from build123d import *

# Parameters (mm, degrees)
SKETCH1_R           = 11
BOSS_EXTRUDE1_DEPTH = 15
SKETCH2_R           = 15
BOSS_EXTRUDE2_DEPTH = 8
SKETCH4_R           = 6.177060042
CUT_EXTRUDE1_DEPTH  = 0.5
SKETCH5_R           = 10
BOSS_EXTRUDE3_DEPTH = 30


with BuildPart() as part:
    # Sketch1 → Boss-Extrude1 (new body)
    with BuildSketch(Plane(origin=(0, 0, 0), x_dir=(1, 0, 0), z_dir=(0, 1, 0))):
        Circle(SKETCH1_R)
    extrude(amount=BOSS_EXTRUDE1_DEPTH)

    # Sketch2 → Boss-Extrude2 (add)
    with BuildSketch(Plane(origin=(0, 15, 0), x_dir=(1, 0, 0), z_dir=(0, 1, 0))):
        Circle(SKETCH2_R)
    extrude(amount=BOSS_EXTRUDE2_DEPTH)

    # Sketch3 → Revolve1 (revolve)
    with BuildSketch(Plane.XY):
        Polygon((-13.565724674, 23.42261725), (-15, 23), (0, 23), (0, 34.488010938), (-7.151825625, 34.488010938), (-8.49615375, 24.916394688), (-8.49615375, 24.638921263), (-13.565724674, 23.145143825), align=None)
    revolve(axis=Axis((0, 31.369169688, 0), (0, -1, 0)))

    # Sketch4 → Cut-Extrude1 (cut)
    with BuildSketch(Plane(origin=(0, 34.488010938, 0), x_dir=(1, 0, 0), z_dir=(0, 1, 0))):
        Circle(SKETCH4_R)
    extrude(amount=-CUT_EXTRUDE1_DEPTH, mode=Mode.SUBTRACT)

    # Sketch5 → Boss-Extrude3 (add)
    with BuildSketch(Plane.XZ):
        Circle(SKETCH5_R)
    extrude(amount=BOSS_EXTRUDE3_DEPTH)


solid = part.part
The listing builds one solid part. Answer for the finished solid, in the listing's coordinates (mm). A direction names the side the tool comes from. Round coordinates to 2 decimals unless told otherwise and drop trailing zeros. Write each loop counter-clockwise with the first axis right and the second up, starting at its lowest first coordinate (ties: lowest second). Pieces come first, ordered by that corner, then holes. Notation, with made-up numbers: (-10, 59) - (16, 59) arc R20 cw to (16, 89) - close; hole circle Ø4 at (-15, -7). An arc over 180 degrees is marked (long way). Use a Markdown table: item, result. Add a question column.
1. Flat-ended cylindrical pins translate along their axes: P1, Ø10, axis at x = -1, z = -1, coming from the +Y side; P2, Ø1.5, axis at x = -2, y = 17.5, coming from the +Z side; P3, Ø6, axis at y = -10.5, z = -10.5, coming from the -X side; P4, Ø3, axis at x = -0.5, y = -19, coming from the -Z side. Find the tip coordinate at first contact, or state that the pin passes through.
2. Consider line 1 (Y direction, x = -6, z = 1); line 2 (X direction, y = 34.1, z = 0); line 3 (X direction, y = -5, z = 0.25). Determine where each line is inside the solid, lowest interval first.
3. The part is cut by section D-D (y = 12). Write down the section's boundary in (x, z).
4. The part is cut by section A-A (x = 0). Write down the section's boundary in (y, z), and give its area (3 significant figures).
5. A tool of negligible diameter and unlimited length cuts with its end or side. For faces 1 (the face through (0, -30, 0)), 2 (the face through (0, 33.988, 0)), 3 (the face through (-2.17, -14.79, -9.76)), from which of +Z, -Z, +X, -X, +Y, -Y can it reach the whole face along a straight path? Write none if from no direction.
6. The part is cut by section C-C (y = -5.5). Write down the section's boundary in (x, z).
7. The part is cut by section B-B (z = 0). Write down the section's boundary in (x, y).
Reported:
| question | item | result |
|---|---|---|
| 1 | P1 | y = 34.49 |
| 1 | P2 | z = 14.95 |
| 1 | P3 | x = -6.61 |
| 1 | P4 | z = -10 |
| 2 | line 1 | -30 to 33.99 |
| 2 | line 2 | -7.21 to -6.18, 6.18 to 7.21 |
| 2 | line 3 | -10 to 10 |
| 3 | outline | circle Ø22 at (0, 0) |
| 4 | outline | (-30, -10) - (0, -10) - (0, -11) - (15, -11) - (15, -15) - (23, -15) - (23.42, -13.57) - (23.15, -13.57) - (24.64, -8.5) - (24.92, -8.5) - (34.49, -7.15) - (34.49, -6.18) - (33.99, -6.18) - (33.99, 6.18) - (34.49, 6.18) - (34.49, 7.15) - (24.92, 8.5) - (24.64, 8.5) - (23.15, 13.57) - (23.42, 13.57) - (23, 15) - (15, 15) - (15, 11) - (0, 11) - (0, 10) - (-30, 10) - close |
| 4 | area | 1,360 mm^2 |
| 5 | face 1 | +Z, -Z, +X, -X, -Y |
| 5 | face 2 | +Y |
| 5 | face 3 | -Y |
| 6 | outline | circle Ø20 at (0, 0) |
| 7 | outline | (-15, 15) - (-11, 15) - (-11, 0) - (-10, 0) - (-10, -30) - (10, -30) - (10, 0) - (11, 0) - (11, 15) - (15, 15) - (15, 23) - (13.57, 23.42) - (13.57, 23.15) - (8.5, 24.64) - (8.5, 24.92) - (7.15, 34.49) - (6.18, 34.49) - (6.18, 33.99) - (-6.18, 33.99) - (-6.18, 34.49) - (-7.15, 34.49) - (-8.5, 24.92) - (-8.5, 24.64) - (-13.57, 23.15) - (-13.57, 23.42) - (-15, 23) - close |
